from build123d import *

# Parameters (mm, degrees)
F0_W     = 17.5
F0_H     = 76
F0_R     = 4
F1_DEPTH = 5
F0_H_2   = 5
F2_DEPTH = 25
F3_R     = 2.5
F4_DEPTH = 100


with BuildPart() as f1:
    # F0 (on Top) → F1 (new body)
    with BuildSketch(Plane.XY):
        Rectangle(F0_W, F0_H)
        with Locations((0, -13)):
            Circle(F0_R, mode=Mode.SUBTRACT)
        with Locations((0, 13)):
            Circle(F0_R, mode=Mode.SUBTRACT)
    extrude(amount=F1_DEPTH)

    # F0 (on Top) → F2 (join)
    with BuildSketch(Plane.XY):
        with Locations((0, 40.5)):
            Rectangle(F0_W, F0_H_2)
        with Locations((0, -40.5)):
            Rectangle(F0_W, F0_H_2)
    extrude(amount=F2_DEPTH)

    # F3 (on face) → F4 (cut)
    with BuildSketch(Plane(origin=(0, 43, 0), x_dir=(-1, 0, 0), z_dir=(0, 1, 0))):
        Polygon((3.75, 25), (8.75, 16), (8.75, 25), align=None)
        Polygon((-8.75, 25), (-8.75, 16), (-3.75, 25), align=None)
        with Locations((0, 19)):
            Circle(F3_R)
    extrude(amount=-F4_DEPTH, mode=Mode.SUBTRACT)


solid = f1.part
Design review of the part built by this model. Coordinates are the model's own, in mm. A direction names the side the tool comes from. Coordinates: 2 decimals unless noted, no trailing zeros. Loops run counter-clockwise (first coordinate to the right, second up) from the corner with the lowest first, then second, coordinate; pieces in that order, holes last. Notation, with made-up numbers: M 89.5,-19.5 L 146.5,-19.5 A22 ccw 146.5,-12.5 Z; hole C 69.25,-20 d11. An arc over 180 degrees is marked long. Use one line per item in the form item = value.
(1) Consider section A-A (x = 0). Write out the cut boundary in (y, z).
Return value:
outline = M -43,0 L -17,0 L -17,5 L -38,5 L -38,16.5 L -43,16.5 Z; M -43,21.5 L -38,21.5 L -38,25 L -43,25 Z; M -9,0 L 9,0 L 9,5 L -9,5 Z; M 17,0 L 43,0 L 43,16.5 L 38,16.5 L 38,5 L 17,5 Z; M 38,21.5 L 43,21.5 L 43,25 L 38,25 Z
(2) Consider section B-B (y = -13). Write out the cut boundary in (x, z), and give its area (3 significant figures).
Return value:
outline = M -8.75,0 L -4,0 L -4,5 L -8.75,5 Z; M 4,0 L 8.75,0 L 8.75,5 L 4,5 Z
area = 47.5 mm2
(3) Consider section D-D (z = 19). Write out the cut boundary in (x, y), and give its area (3 significant figures).
Return value:
outline = M -7.08,-43 L -2.5,-43 L -2.5,-38 L -7.08,-38 Z; M -7.08,38 L -2.5,38 L -2.5,43 L -7.08,43 Z; M 2.5,-43 L 7.08,-43 L 7.08,-38 L 2.5,-38 Z; M 2.5,38 L 7.08,38 L 7.08,43 L 2.5,43 Z
area = 91.7 mm2
(4) For faces 1 (the face through (0, -38, 13)), 2 (the face through (-6.215, 40.535, 20.563)), list the 3-axis set-ups (+Z, -Z, +X, -X, +Y, -Y) from which the entire face can be reached by the end or side of a thin tool; tool diameter is ignored.
Return value:
face_1 = +Z, +X, -X
face_2 = +Z, -X, +Y, -Y
(5) Draft analysis for pull direction Y (two halves, no side actions). For faces 3 (the face through (0, 38, 13)), 4 (the face through (-0.867, -16.905, 2.465)), 5 (the face through (0, -43, 10)), 6 (the face through (-6.215, -40.465, 20.563)), state which applies: pulls with the +Y half, pulls with the -Y half, needs draft (parallel to the pull), parting line crosses it, or undercut.
Return value:
face_3 = undercut
face_4 = undercut
face_5 = pulls with the -Y half
face_6 = needs draft
(6) Consider section C-C (z = 6.5). Write out the cut boundary in (x, y).
Return value:
outline = M -8.75,-43 L 8.75,-43 L 8.75,-38 L -8.75,-38 Z; M -8.75,38 L 8.75,38 L 8.75,43 L -8.75,43 Z
(7) For line 1 along Z through (x, y) = (0, -40.5); line 2 along Y through (x, z) = (-7, 10); line 3 along Z through (x, y) = (-5, 9.5), list the stretches that pass through material, from the lowest coordinate up. Write a range as from..to.
Return value:
line_1 = 0..16.5, 21.5..25
line_2 = -43..-38, 38..43
line_3 = 0..5
(8) Clearance check with flat-ended pins moving along their axes: P1, Ø10, axis at x = 4, y = -23, coming from the +Z side; P2, Ø6.5, axis at x = 0, y = 13, coming from the +Z side; P3, Ø3, axis at x = 2, y = -17, coming from the -Z side. State where each tip first meets the part, or that it passes through.
Return value:
P1 = 5
P2 = through
P3 = 0
